Here's how the part is built. I have some questions about the finished solid (model axes, mm). Face numbers are marked on the shaded views. A direction names the side the tool comes from. Coordinates: 2 decimals unless noted, no trailing zeros. Order: outer loops, then holes, each group sorted by start corner. A loop starts at its lowest first (then second) coordinate and runs counter-clockwise, first axis right, second up. Notation, with made-up numbers: (88, 64) - (116, 64) arc R17 ccw to (116, 91) - close; hole circle Ø9 at (45.5, 82.25). An arc over 180 degrees is marked (long way). Answer in a Markdown table with one row per item. Add a question column.
Item 1: I want a section at D-D (z = -54.5). Please give me the cut outline in (x, y).
Item 2: I want a section at A-A (x = 5.08). Please give me the cut outline in (y, z).
Item 3: On a 3-axis mill with a long thin cutter (end or side, diameter ignored), from which of +Z, -Z, +X, -X, +Y, -Y can I reach the whole of each face in a straight line? I mean the marked faces 5, 6, 7 and 8. Say none if no direction works.
Item 4: Will these pins go through, and if not, where does the flat tip stop? pin 1 Ø6 at (y, z) = (12, -5.5) entering from -X; pin 2 Ø12.5 at (x, z) = (83, -13) entering from +Y; pin 3 Ø3 at (y, z) = (9, 2) entering from -X; pin 4 Ø6 at (y, z) = (15.5, -90.5) entering from -X.
Item 5: If I drill on line 1 along Z through (x, y) = (121.92, 1.3); line 2 along X through (y, z) = (0.8, -121.92); line 3 along X through (y, z) = (13.75, -13) (3 decimals), over which ranges is the centre line in solid material (lowest first)? Write a range as from..to.
Item 6: I want a section at B-B (z = -121.92). Please give me the cut outline in (x, y), plus the area to 3 significant figures.
Item 7: Thinking about a two-plate mould opening in Z: for the marked faces 1, 2, 3 and 4, which applies, +Z half, -Z half, draft (parallel to the pull), parting line (faces both ways), or undercut?
Item 8: I want a section at C-C (y = 21.59). Please give me the cut outline in (x, z) (3 decimals).
```python
from build123d import *

# Parameters (mm, degrees)
SKETCH1_W            = 127
SKETCH1_H            = 127
SKETCH1_R            = 1.5875
BOSS_EXTRUDE1_DEPTH  = 1.778
SKETCH2_W            = 28.194
SKETCH2_H            = 28.575
BOSS_EXTRUDE2_DEPTH  = 2.794
SKETCH3_W            = 10.0584
SKETCH3_H            = 11.6332
BOSS_EXTRUDE3_DEPTH  = 7.366
SKETCH4_W            = 6.35
SKETCH4_H            = 25.4
BOSS_EXTRUDE4_DEPTH  = 11.6078
SKETCH5_W            = 8.763
SKETCH5_H            = 33.02
BOSS_EXTRUDE5_DEPTH  = 9.144
SKETCH6_W            = 10.0584
SKETCH6_H            = 50.292
BOSS_EXTRUDE6_DEPTH  = 6.223
SKETCH7_W            = 4.826
SKETCH7_H            = 8.255
BOSS_EXTRUDE7_DEPTH  = 15.3924
SKETCH8_W            = 7.62
SKETCH8_H            = 5.588
BOSS_EXTRUDE8_DEPTH  = 2.286
SKETCH9_R            = 23.8125
BOSS_EXTRUDE9_DEPTH  = 12.954
SKETCH10_W           = 12.7
SKETCH10_H           = 16.7894
BOSS_EXTRUDE10_DEPTH = 27.432
SKETCH11_R           = 3.4671
BOSS_EXTRUDE11_DEPTH = 3.302
SKETCH12_W           = 15.875
SKETCH12_H           = 21.9202
BOSS_EXTRUDE12_DEPTH = 15.0876
SKETCH13_W           = 5.842
SKETCH13_H           = 25.4
BOSS_EXTRUDE13_DEPTH = 13.716
CHAMFER1_SIZE        = 8.382
SKETCH14_W           = 14.732
SKETCH14_H           = 9.8806
BOSS_EXTRUDE14_DEPTH = 6.096
SKETCH15_W           = 6.604
SKETCH15_H           = 16.9164
BOSS_EXTRUDE15_DEPTH = 8.128
SKETCH16_W           = 30.48
SKETCH16_H           = 12.446
BOSS_EXTRUDE16_DEPTH = 14.351
SKETCH17_W           = 6.35
SKETCH17_H           = 7.8232
CUT_EXTRUDE1_DEPTH   = 8.382
BOSS_EXTRUDE17_DEPTH = 7.112


with BuildPart() as part:
    # Sketch1 → Boss-Extrude1 (new body)
    with BuildSketch(Plane(origin=(0, 0, 0), x_dir=(1, 0, 0), z_dir=(0, 1, 0))):
        with Locations((63.5, 63.5)):
            Rectangle(SKETCH1_W, SKETCH1_H)
        with Locations((5.08, 121.92)):
            Circle(SKETCH1_R, mode=Mode.SUBTRACT)
        with Locations((121.92, 121.92)):
            Circle(SKETCH1_R, mode=Mode.SUBTRACT)
        with Locations((121.92, 5.08)):
            Circle(SKETCH1_R, mode=Mode.SUBTRACT)
        with Locations((5.08, 5.08)):
            Circle(SKETCH1_R, mode=Mode.SUBTRACT)
    extrude(amount=BOSS_EXTRUDE1_DEPTH)

    # Sketch2 → Boss-Extrude2 (add)
    with BuildSketch(Plane(origin=(0, 1.778, 0), x_dir=(1, 0, 0), z_dir=(0, 1, 0))):
        with Locations((31.8262, 112.7125)):
            Rectangle(SKETCH2_W, SKETCH2_H)
    extrude(amount=BOSS_EXTRUDE2_DEPTH)

    # Sketch3 → Boss-Extrude3 (add)
    with BuildSketch(Plane(origin=(0, 1.778, 0), x_dir=(1, 0, 0), z_dir=(0, 1, 0))):
        with Locations((74.4728, 121.1834)):
            Rectangle(SKETCH3_W, SKETCH3_H)
    extrude(amount=BOSS_EXTRUDE3_DEPTH)

    # Sketch4 → Boss-Extrude4 (add)
    with BuildSketch(Plane(origin=(0, 1.778, 0), x_dir=(1, 0, 0), z_dir=(0, 1, 0))):
        with Locations((123.825, 74.422)):
            Rectangle(SKETCH4_W, SKETCH4_H)
    extrude(amount=BOSS_EXTRUDE4_DEPTH)

    # Sketch5 → Boss-Extrude5 (add)
    with BuildSketch(Plane(origin=(0, 1.778, 0), x_dir=(1, 0, 0), z_dir=(0, 1, 0))):
        with Locations((4.3815, 100.33)):
            Rectangle(SKETCH5_W, SKETCH5_H)
    extrude(amount=BOSS_EXTRUDE5_DEPTH)

    # Sketch6 → Boss-Extrude6 (add)
    with BuildSketch(Plane(origin=(0, 1.778, 0), x_dir=(1, 0, 0), z_dir=(0, 1, 0))):
        with Locations((5.0292, 52.9844)):
            Rectangle(SKETCH6_W, SKETCH6_H)
    extrude(amount=BOSS_EXTRUDE6_DEPTH)

    # Sketch7 → Boss-Extrude7 (add)
    with BuildSketch(Plane(origin=(0, 1.778, 0), x_dir=(1, 0, 0), z_dir=(0, 1, 0))):
        with Locations((16.9418, 77.1525)):
            Rectangle(SKETCH7_W, SKETCH7_H)
    extrude(amount=BOSS_EXTRUDE7_DEPTH)

    # Sketch8 → Boss-Extrude8 (add)
    with BuildSketch(Plane(origin=(0, 1.778, 0), x_dir=(1, 0, 0), z_dir=(0, 1, 0))):
        with Locations((112.395, 2.794)):
            Rectangle(SKETCH8_W, SKETCH8_H)
    extrude(amount=BOSS_EXTRUDE8_DEPTH)

    # Sketch9 → Boss-Extrude9 (add)
    with BuildSketch(Plane(origin=(0, 1.778, 0), x_dir=(1, 0, 0), z_dir=(0, 1, 0))):
        with Locations((50.8, 52.07)):
            Circle(SKETCH9_R)
    extrude(amount=BOSS_EXTRUDE9_DEPTH)

    # Sketch10 → Boss-Extrude10 (add)
    with BuildSketch(Plane(origin=(0, 1.778, 0), x_dir=(1, 0, 0), z_dir=(0, 1, 0))):
        with Locations((99.695, 8.3947)):
            Rectangle(SKETCH10_W, SKETCH10_H)
    extrude(amount=BOSS_EXTRUDE10_DEPTH)

    # Sketch11 → Boss-Extrude11 (add)
    with BuildSketch(Plane.XY):
        with Locations((99.695, 21.59)):
            Circle(SKETCH11_R)
        with Locations((99.695, 9.144)):
            Circle(SKETCH11_R)
    extrude(amount=BOSS_EXTRUDE11_DEPTH)

    # Sketch12 → Boss-Extrude12 (add)
    with BuildSketch(Plane(origin=(0, 1.778, 0), x_dir=(1, 0, 0), z_dir=(0, 1, 0))):
        with Locations((82.2325, 9.1821)):
            Rectangle(SKETCH12_W, SKETCH12_H)
    extrude(amount=BOSS_EXTRUDE12_DEPTH)

    # Sketch13 → Boss-Extrude13 (add)
    with BuildSketch(Plane(origin=(0, 1.778, 0), x_dir=(1, 0, 0), z_dir=(0, 1, 0))):
        with Locations((67.691, 12.7)):
            Rectangle(SKETCH13_W, SKETCH13_H)
    extrude(amount=BOSS_EXTRUDE13_DEPTH)

    # Chamfer1
    chamfer1_edges = [part.edges().sort_by_distance(p)[0] for p in [
        (67.691, 15.494, -25.4),
    ]]
    chamfer(chamfer1_edges, length=CHAMFER1_SIZE)

    # Sketch14 → Boss-Extrude14 (add)
    with BuildSketch(Plane(origin=(0, 1.778, 0), x_dir=(1, 0, 0), z_dir=(0, 1, 0))):
        with Locations((50.8, 4.9403)):
            Rectangle(SKETCH14_W, SKETCH14_H)
    extrude(amount=BOSS_EXTRUDE14_DEPTH)

    # Sketch15 → Boss-Extrude15 (add)
    with BuildSketch(Plane(origin=(0, 1.778, 0), x_dir=(1, 0, 0), z_dir=(0, 1, 0))):
        with Locations((88.7222, 42.3418)):
            Rectangle(SKETCH15_W, SKETCH15_H)
    extrude(amount=BOSS_EXTRUDE15_DEPTH)

    # Sketch16 → Boss-Extrude16 (add)
    with BuildSketch(Plane(origin=(0, 1.778, 0), x_dir=(1, 0, 0), z_dir=(0, 1, 0))):
        with Locations((24.638, 6.223)):
            Rectangle(SKETCH16_W, SKETCH16_H)
    extrude(amount=BOSS_EXTRUDE16_DEPTH)

    # Sketch17 → Cut-Extrude1 (cut)
    with BuildSketch(Plane(origin=(0, 16.129, 0), x_dir=(1, 0, 0), z_dir=(0, 1, 0))):
        with Locations((12.573, 8.5344)):
            Rectangle(SKETCH17_W, SKETCH17_H)
        with Locations((36.703, 8.5344)):
            Rectangle(SKETCH17_W, SKETCH17_H)
    extrude(amount=-CUT_EXTRUDE1_DEPTH, mode=Mode.SUBTRACT)

    # Sketch18 → Boss-Extrude17 (add)
    with BuildSketch(Plane.XY):
        Polygon((11.938, 11.4935), (9.738295474, 10.2235), (9.738295474, 7.6835), (11.938, 6.4135), (14.137704526, 7.6835), (14.137704526, 10.2235), align=None)
        Polygon((37.338, 11.4935), (35.138295474, 10.2235), (35.138295474, 7.6835), (37.338, 6.4135), (39.537704526, 7.6835), (39.537704526, 10.2235), align=None)
        with BuildLine():
            Line((17.039926569, 13.665748038), (32.236073431, 13.665748038))
            ThreePointArc((32.236073431, 13.665748038), (33.182386013, 13.242738295), (33.498305774, 12.2555))
            Line((33.498305774, 12.2555), (32.764527996, 5.6515))
            ThreePointArc((32.764527996, 5.6515), (32.34928591, 4.845435455), (31.502295653, 4.521748038))
            Line((31.502295653, 4.521748038), (17.773704347, 4.521748038))
            ThreePointArc((17.773704347, 4.521748038), (16.92671409, 4.845435455), (16.511472004, 5.6515))
            Line((16.511472004, 5.6515), (15.777694226, 12.2555))
            ThreePointArc((15.777694226, 12.2555), (16.093613987, 13.242738295), (17.039926569, 13.665748038))
        make_face()
    extrude(amount=BOSS_EXTRUDE17_DEPTH)


solid = part.part
```
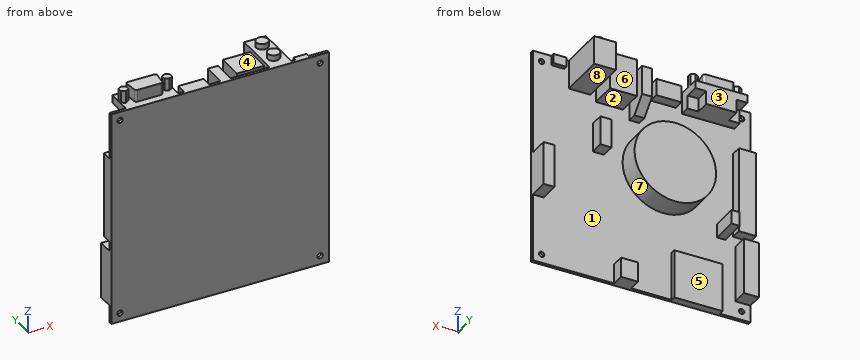
Values follow:
| question | item | result |
|---|---|---|
| 1 | outline | (0, 0) - (127, 0) - (127, 1.78) - (74.49, 1.78) - (74.49, 14.73) - (27.11, 14.73) - (27.11, 1.78) - (10.06, 1.78) - (10.06, 8) - (0, 8) - close |
| 2 | outline | (0, -127) - (1.78, -127) - (1.78, -123.51) - (0, -123.51) - close; (0, -120.33) - (1.78, -120.33) - (1.78, -116.84) - (10.92, -116.84) - (10.92, -83.82) - (1.78, -83.82) - (1.78, -78.13) - (8, -78.13) - (8, -27.84) - (1.78, -27.84) - (1.78, -6.67) - (0, -6.67) - close; (0, -3.49) - (1.78, -3.49) - (1.78, 0) - (0, 0) - close |
| 3 | face 5 | -Z, +Y |
| 3 | face 6 | +Z, -Z, -X, +Y |
| 3 | face 7 | +Y |
| 3 | face 8 | -Z, +X, +Y |
| 4 | pin 1 | stops at x = 9.4 |
| 4 | pin 2 | stops at y = 16.87 |
| 4 | pin 3 | stops at x = 9.74 |
| 4 | pin 4 | passes through |
| 5 | line 1 | z = -127..-123.51, -120.33..-6.67, -3.49..0 |
| 5 | line 2 | x = 0..3.49, 6.67..120.33, 123.51..127 |
| 5 | line 3 | x = 64.77..70.612, 74.295..90.17, 93.345..106.045 |
| 6 | outline | (0, 0) - (3.49, 0) - (3.49, 1.78) - (0, 1.78) - close; (6.67, 0) - (120.33, 0) - (120.33, 1.78) - (79.5, 1.78) - (79.5, 9.14) - (69.44, 9.14) - (69.44, 1.78) - (45.92, 1.78) - (45.92, 4.57) - (17.73, 4.57) - (17.73, 1.78) - (6.67, 1.78) - close; (123.51, 0) - (127, 0) - (127, 1.78) - (123.51, 1.78) - close |
| 6 | area | 367 mm^2 |
| 7 | face 1 | undercut |
| 7 | face 2 | undercut |
| 7 | face 3 | draft |
| 7 | face 4 | +Z half |
| 8 | outline | (93.345, -16.789) - (106.045, -16.789) - (106.045, 0) - (103.162, 0) - (103.162, 3.302) - (96.228, 3.302) - (96.228, 0) - (93.345, 0) - close |
